Work out the finished part from the listing and answer in its coordinate system (mm). Face numbers are marked on the shaded views. Give positions to 0.01 mm unless a question says otherwise; leave off trailing zeros. Write each loop counter-clockwise with the first axis right and the second up, starting at its lowest first coordinate (ties: lowest second). Pieces come first, ordered by that corner, then holes. Notation, with made-up numbers: (40, -14) -> (68, -14) arc R20 cw to (68, -4) -> close; hole circle Ø6 at (81, 61.25). An arc over 180 degrees is marked (long way). Use a Markdown table: item, result. Add a question column.
Q1. Section D-D, the plane y = -4 is taken. Give the vertices of the cut face in (x, z).
Q2. For a pull along X with two mould halves and no side action, classify the marked faces 1, 2 and 3 as pulls with the +X half, pulls with the -X half, needs draft (parallel to the pull), parting line crosses it, or undercut.
Q3. Section A-A, the plane z = 24 is taken. Give the vertices of the cut face in (x, y) (3 decimals), plus the area to 3 significant figures.
Q4. Consider line 1 (Y direction, x = 0, z = 24.5) (3 decimals); line 2 (Y direction, x = 0.5, z = 11.25); line 3 (Z direction, x = 3.5, y = 0.5). Determine where each line is inside the solid, lowest interval first.
Q5. Section B-B, the plane x = 12 is taken. Give the vertices of the cut face in (y, z).
Q6. Section C-C, the plane y = -11 is taken. Give the vertices of the cut face in (x, z), plus the area to 3 significant figures.
Q7. Each of these flat-tipped pins is pushed along its axis until it touches: pin 1 Ø3 at (x, z) = (4, 16) entering from -Y; pin 2 Ø12 at (x, z) = (16, 7.5) entering from -Y; pin 3 Ø12.5 at (x, y) = (9.5, 5) entering from -Z; pin 4 Ø4 at (x, y) = (-10.39, 6) entering from +Z. Where does it stop, or does it pass through?
from build123d import *

# Parameters (mm, degrees)
CROQUIS1_R              = 23
CROQUIS1_R_2            = 21
SALIENTE_EXTRUIR1_DEPTH = 23
CROQUIS2_R              = 23
CROQUIS2_R_2            = 3.125
CROQUIS2_R_3            = 3.5
SALIENTE_EXTRUIR2_DEPTH = 3
CROQUIS3_R              = 21
CROQUIS3_R_2            = 16.5
SALIENTE_EXTRUIR3_DEPTH = 2


with BuildPart() as part:
    # Croquis1 → Saliente-Extruir1 (new body)
    with BuildSketch(Plane.XY):
        Circle(CROQUIS1_R)
        Circle(CROQUIS1_R_2, mode=Mode.SUBTRACT)
    extrude(amount=SALIENTE_EXTRUIR1_DEPTH)

    # Croquis2 → Saliente-Extruir2 (add)
    with BuildSketch(Plane.XY.offset(23)):
        Circle(CROQUIS2_R)
        Circle(CROQUIS2_R_2, mode=Mode.SUBTRACT)
        with Locations((0, 12)):
            Circle(CROQUIS2_R_3, mode=Mode.SUBTRACT)
        with Locations((10.392304845, 6)):
            Circle(CROQUIS2_R_3, mode=Mode.SUBTRACT)
        with Locations((10.392304845, -6)):
            Circle(CROQUIS2_R_3, mode=Mode.SUBTRACT)
        with Locations((0, -12)):
            Circle(CROQUIS2_R_3, mode=Mode.SUBTRACT)
        with Locations((-10.392304845, -6)):
            Circle(CROQUIS2_R_3, mode=Mode.SUBTRACT)
        with Locations((-10.392304845, 6)):
            Circle(CROQUIS2_R_3, mode=Mode.SUBTRACT)
    extrude(amount=SALIENTE_EXTRUIR2_DEPTH)

    # Croquis3 → Saliente-Extruir3 (add)
    with BuildSketch(Plane(origin=(0, 0, 23), x_dir=(-1, 0, 0), z_dir=(0, 0, -1))):
        Circle(CROQUIS3_R)
        Circle(CROQUIS3_R_2, mode=Mode.SUBTRACT)
    extrude(amount=SALIENTE_EXTRUIR3_DEPTH)


solid = part.part
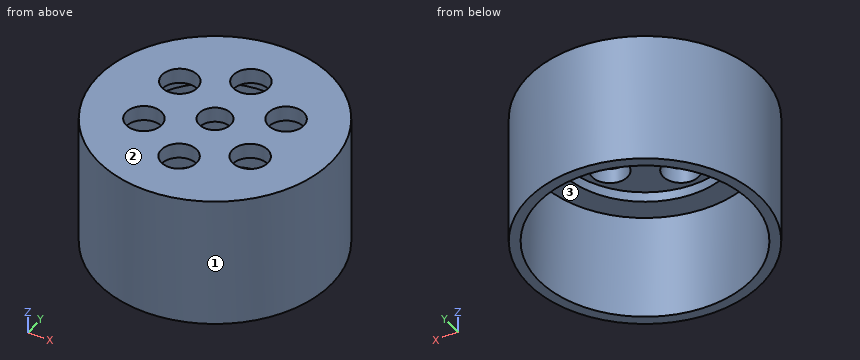
Result set:
| question | item | result |
|---|---|---|
| 1 | outline | (-22.65, 0) -> (-20.62, 0) -> (-20.62, 21) -> (-16.01, 21) -> (-16.01, 23) -> (-13.26, 23) -> (-13.26, 26) -> (-22.65, 26) -> close; (-7.52, 23) -> (7.52, 23) -> (7.52, 26) -> (-7.52, 26) -> close; (13.26, 23) -> (16.01, 23) -> (16.01, 21) -> (20.62, 21) -> (20.62, 0) -> (22.65, 0) -> (22.65, 26) -> (13.26, 26) -> close |
| 2 | face 1 | parting line crosses it |
| 2 | face 2 | needs draft |
| 2 | face 3 | undercut |
| 3 | outline | circle Ø46 at (0, 0); hole circle Ø7 at (-10.392, -6); hole circle Ø7 at (-10.392, 6); hole circle Ø7 at (0, -12); hole circle Ø7 at (0, 12); hole circle Ø6.25 at (0, 0); hole circle Ø7 at (10.392, -6); hole circle Ø7 at (10.392, 6) |
| 3 | area | 1,400 mm2 |
| 4 | line 1 | y = -23 to -15.5, -8.5 to -3.125, 3.125 to 8.5, 15.5 to 23 |
| 4 | line 2 | y = -22.99 to -20.99, 20.99 to 22.99 |
| 4 | line 3 | z = 23 to 26 |
| 5 | outline | (-19.62, 0) -> (-17.23, 0) -> (-17.23, 21) -> (-11.32, 21) -> (-11.32, 23) -> (-9.11, 23) -> (-9.11, 26) -> (-19.62, 26) -> close; (-2.89, 23) -> (2.89, 23) -> (2.89, 26) -> (-2.89, 26) -> close; (9.11, 23) -> (11.32, 23) -> (11.32, 21) -> (17.23, 21) -> (17.23, 0) -> (19.62, 0) -> (19.62, 26) -> (9.11, 26) -> close |
| 6 | outline | (-20.2, 0) -> (-17.89, 0) -> (-17.89, 21) -> (-12.3, 21) -> (-12.3, 23) -> (-3.35, 23) -> (-3.35, 26) -> (-20.2, 26) -> close; (3.35, 23) -> (12.3, 23) -> (12.3, 21) -> (17.89, 21) -> (17.89, 0) -> (20.2, 0) -> (20.2, 26) -> (3.35, 26) -> close |
| 6 | area | 230 mm2 |
| 7 | pin 1 | stops at y = -22.86 |
| 7 | pin 2 | stops at y = -20.71 |
| 7 | pin 3 | stops at z = 21 |
| 7 | pin 4 | passes through |
